Read the model definition and answer for the solid it produces. Units are mm, in the model's axes. Give positions to 0.01 mm unless a question says otherwise; leave off trailing zeros. Loops run counter-clockwise (first coordinate to the right, second up) from the corner with the lowest first, then second, coordinate; pieces in that order, holes last. Notation, with made-up numbers: (82.5, -7) -> (137.5, -7) arc R21 ccw to (137.5, 21) -> close; hole circle Ø1 at (-5, 44.5). An arc over 180 degrees is marked (long way). Write each question's results on one line, items separated by ' | '. Start each with the question number.
Item 1: Find the intervals of material crossed by line 1 (Y direction, x = 16, z = 1.55); line 2 (Y direction, x = 3, z = 0.55); line 3 (X direction, y = 0.5, z = 0.5), in increasing order.
Item 2: Section C-C on y = 4 is taken. Write down the section's boundary in (x, z), and give its area (3 significant figures).
Item 3: Section A-A on y = -16 is taken. Write down the section's boundary in (x, z).
Item 4: Section D-D on y = -7.5 is taken. Write down the section's boundary in (x, z), and give its area (3 significant figures).
Item 5: Each of these flat-tipped pins is pushed along its axis until it touches: P1, Ø8, axis at x = -3.5, y = -9.5, coming from the -Z side; P2, Ø5, axis at x = -16, y = 16, coming from the -Z side. Where does it stop, or does it pass through?
```python
from build123d import *

# Parameters (mm, degrees)
SKETCH_W     = 41
SKETCH_H     = 41
SKETCH_R     = 2
PAD_DEPTH    = 2
FILLET_R     = 0.5
FILLET001_R  = 4
CHAMFER_SIZE = 0.75


with BuildPart() as part:
    # Sketch → Pad (new body)
    with BuildSketch(Plane.XY):
        Rectangle(SKETCH_W, SKETCH_H)
        with Locations((-16, 16)):
            Circle(SKETCH_R, mode=Mode.SUBTRACT)
        with Locations((16, 16)):
            Circle(SKETCH_R, mode=Mode.SUBTRACT)
        with Locations((-16, -16)):
            Circle(SKETCH_R, mode=Mode.SUBTRACT)
        with Locations((16, -16)):
            Circle(SKETCH_R, mode=Mode.SUBTRACT)
        with BuildLine():
            Line((-17.5, 1.2), (-7.960057, 1.2))
            ThreePointArc((-7.960057, 1.2), (-8.05, 0), (-7.960057, -1.2))
            Line((-17.5, -1.2), (-7.960057, -1.2))
            Line((-17.5, -1.2), (-17.5, -11.757359))
            ThreePointArc((-13.781771, -12.084715), (-15.605344, -11.517339), (-17.5, -11.757359))
            Line((-6.477138, -4.780082), (-13.781771, -12.084715))
            ThreePointArc((-6.477138, -4.780082), (-5.69221, -5.69221), (-4.780082, -6.477138))
            Line((-4.780082, -6.477138), (-12.084715, -13.781771))
            ThreePointArc((-11.757359, -17.5), (-11.517339, -15.605344), (-12.084715, -13.781771))
            Line((-11.757359, -17.5), (-1.2, -17.5))
            Line((-1.2, -7.960057), (-1.2, -17.5))
            ThreePointArc((-1.2, -7.960057), (0, -8.05), (1.2, -7.960057))
            Line((1.2, -7.960057), (1.2, -17.5))
            Line((1.2, -17.5), (11.757359, -17.5))
            ThreePointArc((12.084715, -13.781771), (11.517339, -15.605344), (11.757359, -17.5))
            Line((4.780082, -6.477138), (12.084715, -13.781771))
            ThreePointArc((4.780082, -6.477138), (5.69221, -5.69221), (6.477138, -4.780082))
            Line((6.477138, -4.780082), (13.781771, -12.084715))
            ThreePointArc((17.5, -11.757359), (15.605344, -11.517339), (13.781771, -12.084715))
            Line((17.5, -1.2), (17.5, -11.757359))
            Line((7.960057, -1.2), (17.5, -1.2))
            ThreePointArc((7.960057, -1.2), (8.05, 0), (7.960057, 1.2))
            Line((7.960057, 1.2), (17.5, 1.2))
            Line((17.5, 1.2), (17.5, 11.757359))
            ThreePointArc((13.781771, 12.084715), (15.605344, 11.517339), (17.5, 11.757359))
            Line((6.477138, 4.780082), (13.781771, 12.084715))
            ThreePointArc((6.477138, 4.780082), (5.69221, 5.69221), (4.780082, 6.477138))
            Line((4.780082, 6.477138), (12.084715, 13.781771))
            ThreePointArc((11.757359, 17.5), (11.517339, 15.605344), (12.084715, 13.781771))
            Line((1.2, 17.5), (11.757359, 17.5))
            Line((1.2, 7.960057), (1.2, 17.5))
            ThreePointArc((1.2, 7.960057), (0, 8.05), (-1.2, 7.960057))
            Line((-1.2, 7.960057), (-1.2, 17.5))
            Line((-11.757359, 17.5), (-1.2, 17.5))
            ThreePointArc((-12.084715, 13.781771), (-11.517339, 15.605344), (-11.757359, 17.5))
            Line((-4.780082, 6.477138), (-12.084715, 13.781771))
            ThreePointArc((-4.780082, 6.477138), (-5.69221, 5.69221), (-6.477138, 4.780082))
            Line((-6.477138, 4.780082), (-13.781771, 12.084715))
            ThreePointArc((-17.5, 11.757359), (-15.605344, 11.517339), (-13.781771, 12.084715))
            Line((-17.5, 1.2), (-17.5, 11.757359))
        make_face(mode=Mode.SUBTRACT)
    extrude(amount=PAD_DEPTH)

    # Fillet
    fillet_edges = [part.edges().sort_by_distance(p)[0] for p in [
        (-4.780082, -6.477138, 1),
        (-7.960057, -1.2, 1),
        (-7.960057, 1.2, 1),
        (-6.477138, 4.780082, 1),
        (-4.780082, 6.477138, 1),
        (-1.2, 7.960057, 1),
        (1.2, 7.960057, 1),
        (4.780082, 6.477138, 1),
        (6.477138, 4.780082, 1),
        (7.960057, 1.2, 1),
        (7.960057, -1.2, 1),
        (4.780082, -6.477138, 1),
        (-6.477138, -4.780082, 1),
        (-1.2, -7.960057, 1),
        (1.2, -7.960057, 1),
        (6.477138, -4.780082, 1),
    ]]
    fillet(fillet_edges, radius=FILLET_R)

    # Fillet001
    fillet001_edges = [part.edges().sort_by_distance(p)[0] for p in [
        (20.5, -20.5, 1),
        (20.5, 20.5, 1),
        (-20.5, 20.5, 1),
        (-20.5, -20.5, 1),
    ]]
    fillet(fillet001_edges, radius=FILLET001_R)

    # Chamfer
    chamfer_edges = [part.edges().sort_by_distance(p)[0] for p in [
        (14, -16, 0),
        (-18, -16, 0),
        (-18, 16, 0),
        (14, 16, 0),
    ]]
    chamfer(chamfer_edges, length=CHAMFER_SIZE)


solid = part.part
```
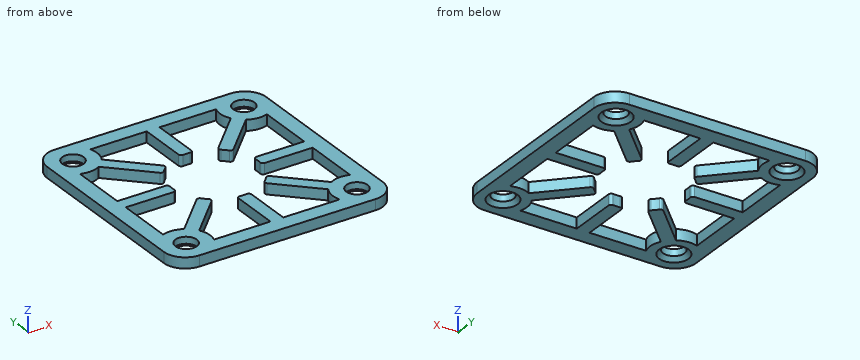
Findings:
1) line 1: -20.5 to -18, -14 to -11.5, -1.2 to 1.2, 11.5 to 14, 18 to 20.5 | line 2: -20.5 to -17.5, 17.5 to 20.5 | line 3: -20.5 to -8.03, 8.03 to 20.5
2) outline: (-20.5, 0) -> (-17.5, 0) -> (-17.5, 2) -> (-20.5, 2) -> close; (17.5, 0) -> (20.5, 0) -> (20.5, 2) -> (17.5, 2) -> close | area: 12.0 mm2
3) outline: (-20.5, 0) -> (-18.75, 0) -> (-18, 0.75) -> (-18, 2) -> (-20.5, 2) -> close; (-14, 0.75) -> (-13.25, 0) -> (-11.5, 0) -> (-11.5, 2) -> (-14, 2) -> close; (-1.2, 0) -> (1.2, 0) -> (1.2, 2) -> (-1.2, 2) -> close; (11.5, 0) -> (13.25, 0) -> (14, 0.75) -> (14, 2) -> (11.5, 2) -> close; (18, 0.75) -> (18.75, 0) -> (20.5, 0) -> (20.5, 2) -> (18, 2) -> close
4) outline: (-20.5, 0) -> (-17.5, 0) -> (-17.5, 2) -> (-20.5, 2) -> close; (-9.2, 0) -> (-5.8, 0) -> (-5.8, 2) -> (-9.2, 2) -> close; (5.8, 0) -> (9.2, 0) -> (9.2, 2) -> (5.8, 2) -> close; (17.5, 0) -> (20.5, 0) -> (20.5, 2) -> (17.5, 2) -> close | area: 25.6 mm2
5) P1: z = 0 | P2: z = 0.25
